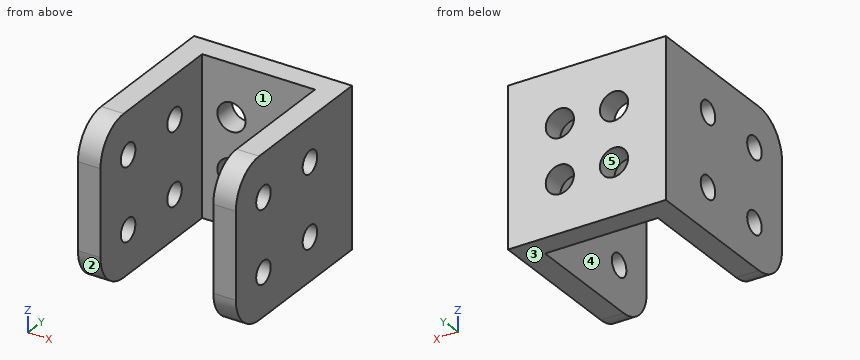
```python
from build123d import *

# Parameters (mm, degrees)
F0_W     = 15.875
F0_H     = 22.225
F0_R     = 1.984375
F1_DEPTH = 3.175
F0_W_2   = 3.175
F2_DEPTH = 25.4
F3_R     = 1.5875
F4_DEPTH = 22.226
F5_R     = 5.08


with BuildPart() as f1:
    # F0 (on Front) → F1 (new body)
    with BuildSketch(Plane.XZ):
        Rectangle(F0_W, F0_H)
        with Locations((-3.81, -3.81)):
            Circle(F0_R, mode=Mode.SUBTRACT)
        with Locations((3.81, -3.81)):
            Circle(F0_R, mode=Mode.SUBTRACT)
        with Locations((-3.81, 3.81)):
            Circle(F0_R, mode=Mode.SUBTRACT)
        with Locations((3.81, 3.81)):
            Circle(F0_R, mode=Mode.SUBTRACT)
    extrude(amount=F1_DEPTH)

    # F0 (on Front) → F2 (join)
    with BuildSketch(Plane.XZ):
        with Locations((9.525, 0)):
            Rectangle(F0_W_2, F0_H)
        with Locations((-9.525, 0)):
            Rectangle(F0_W_2, F0_H)
    extrude(amount=F2_DEPTH)

    # F3 (on face) → F4 (cut, through all)
    with BuildSketch(Plane.YZ.offset(11.1125)):
        with Locations((-19.3675, 5.08)):
            Circle(F3_R)
        with Locations((-9.2075, 5.08)):
            Circle(F3_R)
        with Locations((-9.2075, -5.08)):
            Circle(F3_R)
        with Locations((-19.3675, -5.08)):
            Circle(F3_R)
    extrude(amount=-F4_DEPTH, mode=Mode.SUBTRACT)

    # F5
    f5_edges = [f1.edges().sort_by_distance(p)[0] for p in [
        (9.525, -25.4, 11.1125),
        (-9.525, -25.4, 11.1125),
        (9.525, -25.4, -11.1125),
        (-9.525, -25.4, -11.1125),
    ]]
    fillet(f5_edges, radius=F5_R)


solid = f1.part
```
Source: CAD feature listing. Evaluate the final solid. Frame: model axes, mm. Face numbers are marked on the shaded views. A direction names the side the tool comes from. Coordinates: 2 decimals unless noted, no trailing zeros. Write each loop counter-clockwise with the first axis right and the second up, starting at its lowest first coordinate (ties: lowest second). Pieces come first, ordered by that corner, then holes. Notation, with made-up numbers: (-4.75, 4.5) -> (45.25, 4.5) arc R30 cw to (45.25, 43.5) -> close; hole circle Ø9 at (64.5, -14). An arc over 180 degrees is marked (long way). Return JSON: item names as keys, results as strings. Group by question number.
1) Section query A-A, the plane x = -3.81. Return loops of the section in (y, z) (1 decimal).
2) Section query D-D, the plane z = 2.25. Return loops of the section in (x, y) (1 decimal).
3) Set-up query: the marked faces 1 and 2. Return all of +Z, -Z, +X, -X, +Y, -Y with unobstructed straight access to the full face (end or side cutting, diameter ignored); none if empty.
4) Contact query for flat-ended pins moving along their axis: P1, Ø4, axis at y = -9.21, z = -5.08, coming from the -X side; P2, Ø10, axis at x = 2, z = -6.5, coming from the -Y side (3 decimals). Output: stop coordinate, or through.
5) Section query C-C, the plane z = 0. Return loops of the section in (x, y) (1 decimal).
6) Section query B-B, the plane y = -4.5. Return loops of the section in (x, z), plus the area to 3 significant figures.
7) Ray query, line 1 along Z through (x, y) = (3.81, -1.4); line 2 along Z through (x, y) = (8.5, -19.25); line 3 along X through (y, z) = (-19.5, 7.5). Return the intervals inside material, ascending.
8) Mould query, pull axis Z, two halves, no side actions, for the marked faces 3, 4 and 5. Classes: +Z half, -Z half, draft (parallel to the pull), parting line (faces both ways), or undercut.
From the geometry:
{
 "1": {"outline": "(-3.2, -11.1) -> (0, -11.1) -> (0, -5.8) -> (-3.2, -5.8) -> close; (-3.2, -1.8) -> (0, -1.8) -> (0, 1.8) -> (-3.2, 1.8) -> close; (-3.2, 5.8) -> (0, 5.8) -> (0, 11.1) -> (-3.2, 11.1) -> close"},
 "2": {"outline": "(-11.1, -25.4) -> (-7.9, -25.4) -> (-7.9, -3.2) -> (-5, -3.2) -> (-5, 0) -> (-11.1, 0) -> close; (-2.6, -3.2) -> (2.6, -3.2) -> (2.6, 0) -> (-2.6, 0) -> close; (5, -3.2) -> (7.9, -3.2) -> (7.9, -25.4) -> (11.1, -25.4) -> (11.1, 0) -> (5, 0) -> close"},
 "3": {"face 1": "+Z, -Z, -Y", "face 2": "-Z, +X, -X, -Y"},
 "4": {"P1": "x = -11.11", "P2": "y = -3.175"},
 "5": {"outline": "(-11.1, -25.4) -> (-7.9, -25.4) -> (-7.9, -3.2) -> (7.9, -3.2) -> (7.9, -25.4) -> (11.1, -25.4) -> (11.1, 0) -> (-11.1, 0) -> close"},
 "6": {"outline": "(-11.11, -11.11) -> (-7.94, -11.11) -> (-7.94, 11.11) -> (-11.11, 11.11) -> close; (7.94, -11.11) -> (11.11, -11.11) -> (11.11, 11.11) -> (7.94, 11.11) -> close", "area": "141 mm²"},
 "7": {"line 1": "-11.11 to -5.79, -1.83 to 1.83, 5.79 to 11.11", "line 2": "-11.11 to -6.66, -3.5 to 3.5, 6.66 to 11.11", "line 3": "-11.11 to -7.94, 7.94 to 11.11"},
 "8": {"face 3": "-Z half", "face 4": "draft", "face 5": "undercut"}
}
